Build history of the part. All positions in model axes, mm. Give positions to 0.01 mm unless a question says otherwise; leave off trailing zeros. Order: outer loops, then holes, each group sorted by start corner. A loop starts at its lowest first (then second) coordinate and runs counter-clockwise, first axis right, second up. Notation, with made-up numbers: (2.5, 77.5) - (36.5, 77.5) arc R36 ccw to (36.5, 114.5) - close; hole circle Ø8 at (67, -33.5). An arc over 180 degrees is marked (long way). Use a Markdown table: item, result.
from build123d import *

# Parameters (mm, degrees)
PAD_DEPTH = 2


with BuildPart() as part:
    # Sketch → Pad (new body)
    with BuildSketch(Plane.XY):
        with BuildLine():
            ThreePointArc((25.1, 17.6), (12.55, 18.755091), (0, 17.6))
            Line((0, 24.043957), (0, 17.6))
            ThreePointArc((2.355405, 24.40484), (1.176271, 24.233741), (0, 24.043957))
            ThreePointArc((21.942711, 24.510315), (12.131582, 27.703085), (2.355405, 24.40484))
            ThreePointArc((25.1, 24.043957), (23.523833, 24.293909), (21.942711, 24.510315))
            Line((25.1, 24.043957), (25.1, 17.6))
        make_face()
    extrude(amount=PAD_DEPTH)


solid = part.part
1) Slice it at B-B (y = 25). Write the cut outline in (x, z).
Computed:
| item | result |
|---|---|
| outline | (3.2, 0) - (21.24, 0) - (21.24, 2) - (3.2, 2) - close |
2) Slice it at A-A (z = 1.7). Write the cut outline in (x, y), and give its area (3 significant figures).
Computed:
| item | result |
|---|---|
| outline | (0, 17.6) arc R68.76 cw to (25.1, 17.6) - (25.1, 24.04) arc R75.1 ccw to (21.94, 24.51) arc R16.4 ccw to (2.36, 24.4) arc R75.1 ccw to (0, 24.04) - close |
| area | 195 mm² |
3) Slice it at C-C (x = 23). Write the cut outline in (y, z).
Computed:
| item | result |
|---|---|
| outline | (17.96, 0) - (24.37, 0) - (24.37, 2) - (17.96, 2) - close |
4) Two-plate mould, pull along X, no slides. Class faces 1 (the flat face through (25.1, 21, 1)), 2 (the flat face through (13, 23, 0)), 3 (the flat face through (0, 21, 1)), 4 (the cylindrical face through (12.727, 18.755, 0.986)): +X half, -X half, draft (parallel to the pull), parting line (faces both ways), or undercut.
Computed:
| item | result |
|---|---|
| face 1 | +X half |
| face 2 | draft |
| face 3 | -X half |
| face 4 | undercut |
5) Wall check: line 1 (Y direction, x = 14.25, z = 1.8); line 2 (Y direction, x = 24.25, z = 1); line 3 (X direction, y = 25.75, z = 0.55). Give the ranges that are in metal, low to high. Write a range as from..to.
Computed:
| item | result |
|---|---|
| line 1 | y = 18.73..27.58 |
| line 2 | y = 17.75..24.18 |
| line 3 | x = 4.46..19.98 |
